from build123d import *

# Parameters (mm, degrees)
SKETCH1_R           = 4
BOSS_EXTRUDE1_DEPTH = 8
FILLET1_R           = 10


with BuildPart() as part:
    # Sketch1 → Boss-Extrude1 (new body)
    with BuildSketch(Plane(origin=(0, 0, 0), x_dir=(1, 0, 0), z_dir=(0, 1, 0))):
        Polygon((120, 0), (100, 0), (80, 10), (60, 7), (0, 40), (0, 60), (60, 22), (80, 25), align=None)
        with Locations(Location((60, 15, 0), (0, 0, 270))):
            Circle(SKETCH1_R, mode=Mode.SUBTRACT)
        with Locations(Location((8, 44, 0), (0, 0, 270))):
            Circle(SKETCH1_R, mode=Mode.SUBTRACT)
    extrude(amount=BOSS_EXTRUDE1_DEPTH)

    # Fillet1
    fillet1_edges = [part.edges().sort_by_distance(p)[0] for p in [
        (0, 4, -60),
    ]]
    fillet(fillet1_edges, radius=FILLET1_R)


solid = part.part
Verification items for the finished model (mm, model axes). A direction names the side the tool comes from. Coordinates: 2 decimals unless noted, no trailing zeros. Loops run counter-clockwise (first coordinate to the right, second up) from the corner with the lowest first, then second, coordinate; pieces in that order, holes last. Notation, with made-up numbers: (-31, -2) -> (27, -2) arc R15 ccw to (27, 19) -> close; hole circle Ø2 at (47.5, 56). An arc over 180 degrees is marked (long way). Write each question's results on one line, items separated by ' | '.
Item 1: Tool access check on faces 1 (the face through (90, 4, -5)), 2 (the face through (69.86, 3.94, -23.48)), 3 (the face through (56, 0, -22)). Record the directions out of +Z, -Z, +X, -X, +Y, -Y that give a thin tool (end or side, any length) a straight path to the whole face; none if there is none.
Found:
face 1: +Z, +Y, -Y | face 2: -Z, +Y, -Y | face 3: +Z, -Z, +X, -X, -Y
Item 2: Section check D-D, the plane x = 78. Enter the section's corners in (y, z).
Found:
outline: (0, -24.7) -> (8, -24.7) -> (8, -9.7) -> (0, -9.7) -> close
Item 3: Section check B-B, the plane y = 3.75. Enter the section's corners in (x, z).
Found:
outline: (0, -41.83) arc R10 ccw to (15.35, -50.28) -> (60, -22) -> (80, -25) -> (120, 0) -> (100, 0) -> (80, -10) -> (60, -7) -> (0, -40) -> close; hole circle Ø8 at (8, -44); hole circle Ø8 at (60, -15)
Item 4: Gauge pin test, flat ends, axial feed: pin 1 (3 mm diameter, centred on y = 7, z = -33.5, fed in from -X); pin 2 (10 mm diameter, centred on x = 41.5, z = -16, fed in from -Y); pin 3 (1.5 mm diameter, centred on x = 76, y = 5, fed in from +Z); pin 4 (2 mm diameter, centred on x = 63, y = 2, fed in from +Z). Record the tip position at first contact, or that the pin passes through.
Found:
pin 1: stops at x = 9.09 | pin 2: stops at y = 0 | pin 3: stops at z = -9.29 | pin 4: stops at z = -7.3
Item 5: Material ranges on L1, parallel to X at y = 3.5, z = -15; L2, parallel to X at y = 5, z = -44; L3, parallel to X at y = 3, z = -26, recorded low to high.
Found:
L1: x = 45.45 to 56, 64 to 96 | L2: x = 0.24 to 4, 12 to 25.26 | L3: x = 25.45 to 53.68
Item 6: Section check A-A, the plane z = -15. Enter the section's corners in (x, y).
Found:
outline: (45.45, 0) -> (56, 0) -> (56, 8) -> (45.45, 8) -> close; (64, 0) -> (96, 0) -> (96, 8) -> (64, 8) -> close
Item 7: Mould release check, pull along Z, two halves, no side actions. Record for faces 4 (the face through (5.6, 3.9, -47.2)), 5 (the face through (99.72, 3.944, -12.675)), 6 (the face through (30.42, 3.94, -23.27)): +Z half, -Z half, draft (parallel to the pull), parting line (faces both ways), or undercut.
Found:
face 4: undercut | face 5: -Z half | face 6: +Z half
Item 8: Section check C-C, the plane x = 8. Enter the section's corners in (y, z).
Found:
outline: (0, -51.63) -> (8, -51.63) -> (8, -48) -> (0, -48) -> close; (0, -40) -> (8, -40) -> (8, -35.6) -> (0, -35.6) -> close
